```python
from build123d import *

# Parameters (mm, degrees)
SKETCH1_W           = 10
SKETCH1_H           = 16
BOSS_EXTRUDE1_DEPTH = 12
SKETCH2_W           = 7
SKETCH2_H           = 10
CUT_EXTRUDE1_DEPTH  = 19.01714389
CUT_EXTRUDE2_DEPTH  = 17.615986871
CUT_EXTRUDE3_DEPTH  = 3.0448
SKETCH4_W           = 4.1
SKETCH4_H           = 6.3
CUT_EXTRUDE4_DEPTH  = 17.022125129
FILLET2_R           = 1
CUT_EXTRUDE7_DEPTH  = 3


with BuildPart() as part:
    # Sketch1 → Boss-Extrude1 (new body)
    with BuildSketch(Plane(origin=(0, 0, 0), x_dir=(0, 0, -1), z_dir=(1, 0, 0))):
        with Locations((0.664893617, 0.978723404)):
            Rectangle(SKETCH1_W, SKETCH1_H)
    extrude(amount=BOSS_EXTRUDE1_DEPTH)

    # Sketch2 → Cut-Extrude1 (cut, through all)
    with BuildSketch(Plane.XY.offset(4.335106383)):
        with Locations((8.5, 3.978723404)):
            Rectangle(SKETCH2_W, SKETCH2_H)
    extrude(amount=-CUT_EXTRUDE1_DEPTH, mode=Mode.SUBTRACT)

    # Sketch3 → Cut-Extrude2 (cut, through all)
    with BuildSketch(Plane(origin=(0, -1.021276596, 0), x_dir=(1, 0, 0), z_dir=(0, 1, 0))):
        with BuildLine():
            ThreePointArc((7.75, 2.254893617), (6.625700218, 1.789193399), (6.16, 0.664893617))
            Line((6.16, 0.664893617), (10.84, 0.664893617))
            ThreePointArc((10.84, 0.664893617), (10.374299782, 1.789193399), (9.25, 2.254893617))
            Line((9.25, 2.254893617), (7.75, 2.254893617))
        make_face()
        with BuildLine():
            Line((10.84, 0.664893617), (6.16, 0.664893617))
            ThreePointArc((6.16, 0.664893617), (6.625700218, -0.459406165), (7.75, -0.925106383))
            Line((7.75, -0.925106383), (9.25, -0.925106383))
            ThreePointArc((9.25, -0.925106383), (10.374299782, -0.459406165), (10.84, 0.664893617))
        make_face()
    extrude(amount=-CUT_EXTRUDE2_DEPTH, mode=Mode.SUBTRACT)

    # Sketch3_3 → Cut-Extrude3 (cut)
    with BuildSketch(Plane(origin=(0, -1.021276596, 0), x_dir=(1, 0, 0), z_dir=(0, 1, 0))):
        with BuildLine():
            ThreePointArc((7.75, 3.138993617), (6.000547113, 2.414346504), (5.2759, 0.664893617))
            Line((5.2759, 0.664893617), (6.16, 0.664893617))
            ThreePointArc((6.16, 0.664893617), (6.625700218, 1.789193399), (7.75, 2.254893617))
            Line((7.75, 2.254893617), (9.25, 2.254893617))
            ThreePointArc((9.25, 2.254893617), (10.374299782, 1.789193399), (10.84, 0.664893617))
            Line((10.84, 0.664893617), (11.7241, 0.664893617))
            ThreePointArc((11.7241, 0.664893617), (10.999452887, 2.414346504), (9.25, 3.138993617))
            Line((9.25, 3.138993617), (7.75, 3.138993617))
        make_face()
        with BuildLine():
            Line((6.16, 0.664893617), (5.2759, 0.664893617))
            ThreePointArc((5.2759, 0.664893617), (6.000547113, -1.08455927), (7.75, -1.809206383))
            Line((7.75, -1.809206383), (9.25, -1.809206383))
            ThreePointArc((9.25, -1.809206383), (10.999452887, -1.08455927), (11.7241, 0.664893617))
            Line((11.7241, 0.664893617), (10.84, 0.664893617))
            ThreePointArc((10.84, 0.664893617), (10.374299782, -0.459406165), (9.25, -0.925106383))
            Line((9.25, -0.925106383), (7.75, -0.925106383))
            ThreePointArc((7.75, -0.925106383), (6.625700218, -0.459406165), (6.16, 0.664893617))
        make_face()
    extrude(amount=-CUT_EXTRUDE3_DEPTH, mode=Mode.SUBTRACT)

    # Sketch4 → Cut-Extrude4 (cut, through all)
    with BuildSketch(Plane.ZY):
        with Locations((-0.664893617, 3.128723404)):
            Rectangle(SKETCH4_W, SKETCH4_H)
    extrude(amount=-CUT_EXTRUDE4_DEPTH, mode=Mode.SUBTRACT)

    # Fillet2
    fillet2_edges = [part.edges().sort_by_distance(p)[0] for p in [
        (2.5, -0.021276596, -2.714893617),
        (2.5, 6.278723404, -2.714893617),
        (2.5, 6.278723404, 1.385106383),
        (2.5, -0.021276596, 1.385106383),
    ]]
    fillet(fillet2_edges, radius=FILLET2_R)

    # Sketch4_6 → Cut-Extrude7 (cut)
    with BuildSketch(Plane.ZY):
        with BuildLine():
            Line((1.385106383, 8.978723404), (-2.714893617, 8.978723404))
            Line((-2.714893617, 8.978723404), (-2.714893617, 5.278723404))
            ThreePointArc((-2.714893617, 5.278723404), (-2.422000398, 5.985830185), (-1.714893617, 6.278723404))
            Line((-1.714893617, 6.278723404), (0.385106383, 6.278723404))
            ThreePointArc((0.385106383, 6.278723404), (1.092213164, 5.985830185), (1.385106383, 5.278723404))
            Line((1.385106383, 5.278723404), (1.385106383, 8.978723404))
        make_face()
        with BuildLine():
            ThreePointArc((-1.714893617, -0.021276596), (-2.422000398, 0.271616623), (-2.714893617, 0.978723404))
            Line((-2.714893617, 0.978723404), (-2.714893617, -0.946152887))
            Line((-2.714893617, -0.946152887), (1.385106383, -0.946152887))
            Line((1.385106383, -0.946152887), (1.385106383, 0.978723404))
            ThreePointArc((1.385106383, 0.978723404), (1.092213164, 0.271616623), (0.385106383, -0.021276596))
            Line((0.385106383, -0.021276596), (-1.714893617, -0.021276596))
        make_face()
    extrude(amount=-CUT_EXTRUDE7_DEPTH, mode=Mode.SUBTRACT)


solid = part.part
```
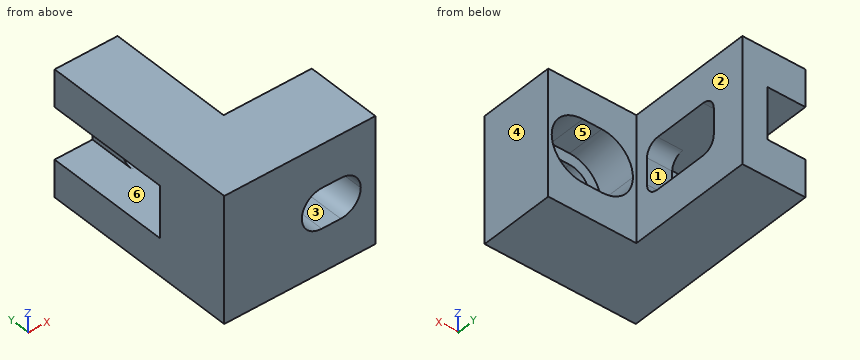
Here's how the part is built. I have some questions about the finished solid (model axes, mm). Face numbers are marked on the shaded views. A direction names the side the tool comes from. Coordinates: 2 decimals unless noted, no trailing zeros. Order: outer loops, then holes, each group sorted by start corner. A loop starts at its lowest first (then second) coordinate and runs counter-clockwise, first axis right, second up.
1) Which directions (+Z, -Z, +X, -X, +Y, -Y) give clear straight access to the entire face, cutting with the end or side of a thin tool? Please do the marked faces 1, 2 and 3.
2) We'd pull the mould along X, two halves only. Please class the marked faces 4, 5 and 6: +X half, -X half, draft (parallel to the pull), parting line (faces both ways), or undercut.
3) Will these pins go through, and if not, where does the flat tip stop? pin 1 (0.6 mm diameter, centred on y = -0.5, z = -1, fed in from -X); pin 2 (5 mm diameter, centred on x = 9, z = -2, fed in from +Y); pin 3 (1.5 mm diameter, centred on x = 1.5, z = 0, fed in from +Y).
4) Imagine slicing it at A-A on y = -1.75. List the corners of the cut face in (x, z) for me.
5) Imagine slicing it at C-C on y = 2. List the corners of the cut face in (x, z) for me.
6) Imagine slicing it at D-D on x = 4.75. List the corners of the cut face in (y, z) for me, and give its area (3 significant figures).
7) I need wall thicknesses on line 1 (Z direction, x = 2.25, y = 7.25); line 2 (Z direction, x = 8, y = -5.75); line 3 (Y direction, x = 7.75, z = 3). Which ranges of each line are inside material? Lowest first, please.
8) Imagine slicing it at B-B on x = 10.25. List the corners of the cut face in (y, z) for me.
Response values:
1. face 1: +X, -X
1. face 2: +Z, -Z, +X, +Y
1. face 3: +Y, -Y
2. face 4: +X half
2. face 5: undercut
2. face 6: draft
3. pin 1: stops at x = 3
3. pin 2: stops at y = -1.02
3. pin 3: stops at y = -0.95
4. outline: (0, -5.66) - (12, -5.66) - (12, 4.34) - (0, 4.34) - close; hole (7.75, -3.14) - (9.25, -3.14) arc R2.47 ccw to (9.25, 1.81) - (7.75, 1.81) arc R2.47 ccw to start
5. outline: (0, -5.66) - (5, -5.66) - (5, -2.71) - (0, -2.71) - close; (0, 1.39) - (5, 1.39) - (5, 4.34) - (0, 4.34) - close
6. outline: (-7.02, -5.66) - (8.98, -5.66) - (8.98, 4.34) - (-7.02, 4.34) - close; hole (-0.02, -1.71) arc R1 ccw to (0.98, -2.71) - (5.28, -2.71) arc R1 ccw to (6.28, -1.71) - (6.28, 0.39) arc R1 ccw to (5.28, 1.39) - (0.98, 1.39) arc R1 ccw to (-0.02, 0.39) - close
6. area: 135 mm2
7. line 1: z = -5.66 to -2.71, 1.39 to 4.34
7. line 2: z = -5.66 to -2.25, 0.93 to 4.34
7. line 3: y = -7.02 to -1.02
8. outline: (-7.02, -5.66) - (-1.02, -5.66) - (-1.02, -2.93) - (-4.07, -2.93) - (-4.07, -1.9) - (-7.02, -1.9) - close; (-7.02, 0.57) - (-4.07, 0.57) - (-4.07, 1.6) - (-1.02, 1.6) - (-1.02, 4.34) - (-7.02, 4.34) - close
